from build123d import *

# Parameters (mm, degrees)
F1_DEPTH = 205
F2_R     = 1
F3_T     = -0.8


with BuildPart() as f1:
    # F0 (on Front) → F1 (new body)
    with BuildSketch(Plane.XZ):
        with BuildLine():
            Line((0, 0), (-12, 0))
            ThreePointArc((-12, 0), (-11.122366, -4.504771), (-8.617839, -8.35062))
            Line((-8.617839, -8.35062), (0, 0))
        make_face()
    extrude(amount=F1_DEPTH)

    # F2
    f2_edges = [f1.edges().sort_by_distance(p)[0] for p in [
        (-8.617839, -102.5, -8.35062),
        (-4.30892, -205, -4.17531),
        (-11.122366, -205, -4.504771),
        (-4.30892, 0, -4.17531),
        (-11.122366, 0, -4.504771),
    ]]
    fillet(f2_edges, radius=F2_R)

    # F3
    f3_openings = [f1.faces().sort_by_distance(p)[0] for p in [
        (-6.000416, -102.5, 0),
    ]]
    offset(amount=F3_T, openings=f3_openings)


solid = f1.part
Build history of the part. All positions in model axes, mm. A direction names the side the tool comes from. Coordinates: 2 decimals unless noted, no trailing zeros. Write each loop counter-clockwise with the first axis right and the second up, starting at its lowest first coordinate (ties: lowest second). Pieces come first, ordered by that corner, then holes.
(1) Mould opens along X. For faces 3 (the cylindrical face through (-11.335, -101.079, -3.94)), 4 (the flat face through (-7, -0.8, -3)), 5 (the flat face through (-0.6, -102, 0)) say: pulls with the +X half, pulls with the -X half, needs draft (parallel to the pull), parting line crosses it, or undercut.
(2) 3-axis set-ups, long thin cutter, end or side, ignore diameter. For faces 1 (the cylindrical face through (-4.775, -204.14, -3.434)), 2 (the flat face through (-7, -205, -3)): which of +Z, -Z, +X, -X, +Y, -Y reach the whole face in a straight line?
(3) Pin check, flat tips, straight feed: pin 1 Ø5 at (x, y) = (-6, -112) entering from +Z; pin 2 Ø3 at (x, z) = (-3.5, -4.5) entering from +Y; pin 3 Ø2 at (x, y) = (-8.5, -110) entering from +Z. Stop position of each tip, or through.
(4) Drill centre lines: line 1 (Y direction, x = -10.75, z = -1.75); line 2 (X direction, y = -50, z = -1.75); line 3 (X direction, y = -58, z = -4.25). Where is each one in solid material? Low to high.
(5) Cut at A-A on y = -60. List the corners of the cut face in (x, z), and give its area (3 significant figures).
Working result:
1. face 3: pulls with the -X half
1. face 4: undercut
1. face 5: needs draft
2. face 1: +Z
2. face 2: +Z, -Z, +X, -X, -Y
3. pin 1: stops at z = -2.28
3. pin 2: stops at y = -0.04
3. pin 3: stops at z = -5.93
4. line 1: y = -205 to -204.2, -0.8 to 0
4. line 2: x = -11.87 to -11.06, -2.96 to -1.81
4. line 3: x = -11.22 to -10.36, -5.54 to -4.39
5. outline: (-12, 0) arc R12 ccw to (-9.34, -7.53) arc R1 ccw to (-7.87, -7.62) - (0, 0) - (-1.15, 0) - (-8.42, -7.05) arc R0.2 cw to (-8.72, -7.03) arc R11.2 cw to (-11.2, 0) - close
5. area: 15.5 mm2
